```python
from build123d import *

# Parameters (mm, degrees)
SKETCH_1_W          = 46
SKETCH_1_H          = 20
SKETCH_1_R          = 1.6
EXTRUDE_1_DEPTH     = 6.5
SKETCH_2_W          = 29.5
SKETCH_2_H          = 10
CUT_EXTRUDE_1_DEPTH = 0.25
SKETCH_3_R          = 2
CUT_EXTRUDE_2_DEPTH = 5.3
SKETCH_4_R          = 1.35
CUT_EXTRUDE_3_DEPTH = 1
SKETCH_5_W          = 11.5
SKETCH_5_H          = 6
CUT_EXTRUDE_4_DEPTH = 5
SKETCH_7_W          = 6.5
SKETCH_7_H          = 5
CUT_EXTRUDE_5_DEPTH = 48.521047968


with BuildPart() as part:
    # 草图1 → 凸台-拉伸1 (new body)
    with BuildSketch(Plane(origin=(0, 0, 0), x_dir=(1, 0, 0), z_dir=(0, 1, 0))):
        Rectangle(SKETCH_1_W, SKETCH_1_H)
        with Locations(Location((-19.5, 7, 0), (0, 0, 90))):
            Circle(SKETCH_1_R, mode=Mode.SUBTRACT)
        with Locations(Location((19.5, 7, 0), (0, 0, 90))):
            Circle(SKETCH_1_R, mode=Mode.SUBTRACT)
        with Locations(Location((-19.5, -7, 0), (0, 0, 90))):
            Circle(SKETCH_1_R, mode=Mode.SUBTRACT)
        with Locations(Location((19.5, -7, 0), (0, 0, 90))):
            Circle(SKETCH_1_R, mode=Mode.SUBTRACT)
    extrude(amount=EXTRUDE_1_DEPTH)

    # 草图2 → 切除-拉伸1 (cut)
    with BuildSketch(Plane(origin=(0, 6.5, 0), x_dir=(1, 0, 0), z_dir=(0, 1, 0))):
        with Locations((8.25, 0)):
            Rectangle(SKETCH_2_W, SKETCH_2_H)
    extrude(amount=-CUT_EXTRUDE_1_DEPTH, mode=Mode.SUBTRACT)

    # 草图3 → 切除-拉伸2 (cut)
    with BuildSketch(Plane(origin=(0, 6.25, 0), x_dir=(1, 0, 0), z_dir=(0, 1, 0))):
        with Locations(Location((-1.5, 0, 0), (0, 0, 270))):
            Circle(SKETCH_3_R)
    extrude(amount=-CUT_EXTRUDE_2_DEPTH, mode=Mode.SUBTRACT)

    # 草图4 → 切除-拉伸3 (cut)
    with BuildSketch(Plane(origin=(0, 0.95, 0), x_dir=(1, 0, 0), z_dir=(0, 1, 0))):
        with Locations(Location((-1.5, 0, 0), (0, 0, 270))):
            Circle(SKETCH_4_R)
    extrude(amount=-CUT_EXTRUDE_3_DEPTH, mode=Mode.SUBTRACT)

    # 草图5 → 切除-拉伸4 (cut)
    with BuildSketch(Plane(origin=(0, 6.25, 0), x_dir=(1, 0, 0), z_dir=(0, 1, 0))):
        with Locations((17.25, 0)):
            Rectangle(SKETCH_5_W, SKETCH_5_H)
    extrude(amount=-CUT_EXTRUDE_4_DEPTH, mode=Mode.SUBTRACT)

    # 草图7 → 切除-拉伸5 (cut, through all)
    with BuildSketch(Plane(origin=(23, 0, 0), x_dir=(0, 0, -1), z_dir=(1, 0, 0))):
        with Locations((-6.75, 2.5)):
            Rectangle(SKETCH_7_W, SKETCH_7_H)
        with Locations((6.75, 2.5)):
            Rectangle(SKETCH_7_W, SKETCH_7_H)
    extrude(amount=-CUT_EXTRUDE_5_DEPTH, mode=Mode.SUBTRACT)


solid = part.part
```
Here's how the part is built. I have some questions about the finished solid (model axes, mm). A direction names the side the tool comes from. Coordinates: 2 decimals unless noted, no trailing zeros. Order: outer loops, then holes, each group sorted by start corner. A loop starts at its lowest first (then second) coordinate and runs counter-clockwise, first axis right, second up.
1) Will these pins go through, and if not, where does the flat tip stop? pin 1 (1 mm diameter, centred on x = -13.5, y = 0.5, fed in from -Z); pin 2 (10 mm diameter, centred on x = 13.5, z = -5, fed in from -Y); pin 3 (3 mm diameter, centred on y = 2, z = 7, fed in from +X); pin 4 (2 mm diameter, centred on x = -11, z = 7, fed in from -Y).
2) Which directions (+Z, -Z, +X, -X, +Y, -Y) give clear straight access to the entire face, cutting with the end or side of a thin tool? Please do faces 1 (the face through (0, 5, -7)), 2 (the face through (-2.7, 3.6, -1.6)), 3 (the face through (11.5, 4, 0)).
3) Imagine slicing it at A-A on z = 0. List the corners of the cut face in (x, y) for me.
4) Imagine slicing it at B-B on x = -1.5. List the corners of the cut face in (y, z) for me, and give its area (3 significant figures).
5) I need wall thicknesses on line 1 (X direction, y = 6.25, z = 7); line 2 (Z direction, x = 19.5, y = 5.4); line 3 (X direction, y = 0.2, z = 0). Which ranges of each line are inside material? Lowest first, please.
6) We'd pull the mould along Z, two halves only. Please class faces 4 (the face through (-23, 4, 0)), 5 (the face through (0, 6, -10)), 6 (the face through (17.914, 5.74, -6.792)): +Z half, -Z half, draft (parallel to the pull), parting line (faces both ways), or undercut.
7) Imagine slicing it at C-C on y = 5.5. List the corners of the cut face in (x, z) for me, and give its area (3 significant figures).
8) Imagine slicing it at D-D on z = -7. List the corners of the cut face in (x, y) for me.
Response values:
1. pin 1: stops at z = -3.5
1. pin 2: stops at y = 0
1. pin 3: passes through
1. pin 4: stops at y = 5
2. face 1: -Z, +X, -X, -Y
2. face 2: +Y
2. face 3: +X, +Y
3. outline: (-23, 0) - (-2.85, 0) - (-2.85, 0.95) - (-3.5, 0.95) - (-3.5, 6.25) - (-6.5, 6.25) - (-6.5, 6.5) - (-23, 6.5) - close; (-0.15, 0) - (23, 0) - (23, 1.25) - (11.5, 1.25) - (11.5, 6.25) - (0.5, 6.25) - (0.5, 0.95) - (-0.15, 0.95) - close
4. outline: (0, -3.5) - (5, -3.5) - (5, -10) - (6.5, -10) - (6.5, -5) - (6.25, -5) - (6.25, -2) - (0.95, -2) - (0.95, -1.35) - (0, -1.35) - close; (0, 1.35) - (0.95, 1.35) - (0.95, 2) - (6.25, 2) - (6.25, 5) - (6.5, 5) - (6.5, 10) - (5, 10) - (5, 3.5) - (0, 3.5) - close
4. area: 38.7 mm2
5. line 1: x = -23 to -21.1, -17.9 to 17.9, 21.1 to 23
5. line 2: z = -10 to -8.6, -5.4 to -3, 3 to 5.4, 8.6 to 10
5. line 3: x = -23 to -2.85, -0.15 to 23
6. face 4: draft
6. face 5: -Z half
6. face 6: undercut
7. outline: (-23, -10) - (23, -10) - (23, -3) - (11.5, -3) - (11.5, 3) - (23, 3) - (23, 10) - (-23, 10) - close; hole circle Ø3.2 at (-19.5, -7); hole circle Ø3.2 at (-19.5, 7); hole circle Ø4 at (-1.5, 0); hole circle Ø3.2 at (19.5, -7); hole circle Ø3.2 at (19.5, 7)
7. area: 806 mm2
8. outline: (-23, 5) - (-21.1, 5) - (-21.1, 6.5) - (-23, 6.5) - close; (-17.9, 5) - (17.9, 5) - (17.9, 6.5) - (-17.9, 6.5) - close; (21.1, 5) - (23, 5) - (23, 6.5) - (21.1, 6.5) - close
